```python
from build123d import *

# Parameters (mm, degrees)
SKETCH1_W           = 140
SKETCH1_H           = 120
SKETCH1_W_2         = 136
SKETCH1_H_2         = 111
BOSS_EXTRUDE1_DEPTH = 16
SKETCH2_R           = 1.25
CUT_EXTRUDE1_DEPTH  = 140.842768851


with BuildPart() as part:
    # Sketch1 → Boss-Extrude1 (new body)
    # profile 1 of 2: a face of its own
    with BuildSketch(Plane(origin=(0, 0, 0), x_dir=(1, 0, 0), z_dir=(0, 1, 0))):
        Rectangle(SKETCH1_W, SKETCH1_H)
        Rectangle(SKETCH1_W_2, SKETCH1_H_2, mode=Mode.SUBTRACT)
    # profile 2 of 2: a face of its own
    with BuildSketch(Plane(origin=(0, 0, 0), x_dir=(1, 0, 0), z_dir=(0, 1, 0))):
        Polygon((-1.273083994, 0), (-45, -55.5), (-42.453832012, -55.5), (0, -1.615850559), (42.453832012, -55.5), (45, -55.5), (1.273083994, 0), (45, 55.5), (42.453832012, 55.5), (0, 1.615850559), (-42.453832012, 55.5), (-45, 55.5), align=None)
    extrude(amount=BOSS_EXTRUDE1_DEPTH)

    # Sketch2 → Cut-Extrude1 (cut, through all)
    with BuildSketch(Plane.XY.offset(60)):
        with BuildLine():
            ThreePointArc((-55.15, 8), (-57.15, 10), (-59.15, 8))
            Line((-59.15, 8), (-59.15, 0))
            Line((-59.15, 0), (-55.15, 0))
            Line((-55.15, 0), (-55.15, 8))
        make_face()
        with Locations((-51.65, 8)):
            Circle(SKETCH2_R)
        with Locations((-62.65, 8)):
            Circle(SKETCH2_R)
        with BuildLine():
            Line((55.15, 8), (55.15, 0))
            Line((55.15, 0), (59.15, 0))
            Line((59.15, 0), (59.15, 8))
            ThreePointArc((59.15, 8), (57.15, 10), (55.15, 8))
        make_face()
        with Locations((51.65, 8)):
            Circle(SKETCH2_R)
        with Locations((62.65, 8)):
            Circle(SKETCH2_R)
    extrude(amount=-CUT_EXTRUDE1_DEPTH, mode=Mode.SUBTRACT)


solid = part.part
```
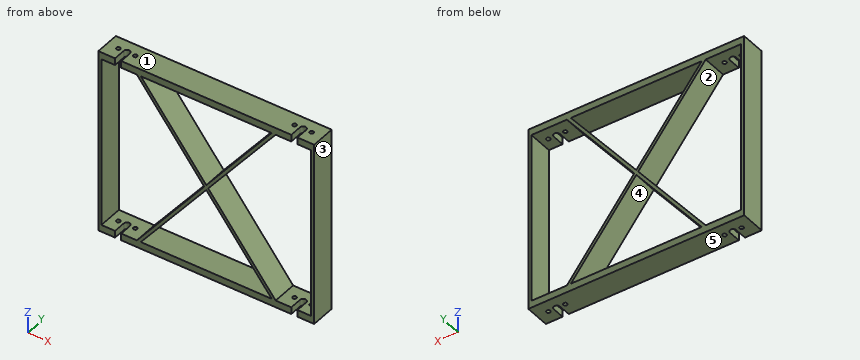
Work out the finished part from the listing and answer in its coordinate system (mm). Face numbers are marked on the shaded views. A direction names the side the tool comes from. Give positions to 0.01 mm unless a question says otherwise; leave off trailing zeros. Loops run counter-clockwise (first coordinate to the right, second up) from the corner with the lowest first, then second, coordinate; pieces in that order, holes last. Notation, with made-up numbers: (-14.5, 21) -> (3.5, 21) arc R30 ccw to (3.5, 56) -> close; hole circle Ø7 at (80, 85). An arc over 180 degrees is marked (long way). Put each result on its own line as item: value. Start each with the question number.
Item 1: The mould has two halves that part along Z. Classify the marked faces 3, 4 and 5: released by +Z, released by -Z, zero draft, split by the parting line, or undercut.
Item 2: Which of the six approach directions +Z, -Z, +X, -X, +Y, -Y give full straight-line access (tool end or side, diameter ignored) to the marked faces 1 and 2?
Item 3: The part is cut by section A-A (x = 57.15). Give the vertices of the cut face in (y, z), then the cut area to 3 significant figures.
Item 4: This flat-tipped pin is pushed along its axis until it touches: P1, Ø3, axis at x = -62.65, y = 8, coming from the -Z side. Where does it stop, or does it pass through?
Item 5: The part is cut by section B-B (z = -24). Give the vertices of the cut face in (x, y), then the cut area to 3 significant figures.
Item 6: Find the intervals of material crossed by L1, parallel to Z at x = 50, y = 0.5; L2, parallel to X at y = 13.75, z = 10.5; L3, parallel to X at y = 14, z = 1.5, in increasing order. Write a range as [from, to].
Answers below:
1. face 3: zero draft
1. face 4: undercut
1. face 5: released by -Z
2. face 1: +Z, +X, -X, +Y, -Y
2. face 2: +Y, -Y
3. outline: (10, -60) -> (16, -60) -> (16, -55.5) -> (10, -55.5) -> close; (10, 55.5) -> (16, 55.5) -> (16, 60) -> (10, 60) -> close
3. area: 54.0 mm2
4. P1: z = -60
5. outline: (-70, 0) -> (-68, 0) -> (-68, 16) -> (-70, 16) -> close; (-20.18, 0) -> (-17.64, 0) -> (-17.64, 16) -> (-20.18, 16) -> close; (17.64, 0) -> (20.18, 0) -> (20.18, 16) -> (17.64, 16) -> close; (68, 0) -> (70, 0) -> (70, 16) -> (68, 16) -> close
5. area: 145 mm2
6. L1: [-60, -55.5], [55.5, 60]
6. L2: [-70, -68], [-9.55, -7], [7, 9.55], [68, 70]
6. L3: [-70, -68], [-2.45, 2.45], [68, 70]
